```python
from build123d import *

# Parameters (mm, degrees)
F0_W     = 22.225
F0_H     = 63.5
F3_D     = 10.16
F2_R     = 19.682221
F4_DEPTH = 61.468


with BuildPart() as f1:
    # F0 (on Front) → F1 (revolve)
    with BuildSketch(Plane.XZ):
        with Locations((-11.1125, 0)):
            Rectangle(F0_W, F0_H)
    revolve(axis=Axis((0, 0, 0), (0, 0, -1)))

    # F3 (through all)
    with Locations(Plane.XY.offset(31.75)):
        with Locations((0, 0)):
            Hole(F3_D / 2)

    # F2 (on face) → F4 (cut)
    with BuildSketch(Plane.XY.offset(31.75)):
        Circle(F2_R)
    extrude(amount=-F4_DEPTH, mode=Mode.SUBTRACT)


solid = f1.part
```
Here's how the part is built. I have some questions about the finished solid (model axes, mm). A direction names the side the tool comes from. Round coordinates to 2 decimals unless told otherwise and drop trailing zeros. Loops run counter-clockwise (first coordinate to the right, second up) from the corner with the lowest first, then second, coordinate; pieces in that order, holes last.
1. Will these pins go through, and if not, where does the flat tip stop? pin 1 (8 mm diameter, centred on x = 12, z = -20, fed in from +Y); pin 2 (4 mm diameter, centred on y = -15.5, z = 18, fed in from -X); pin 3 (5 mm diameter, centred on x = 4.5, z = 2.5, fed in from -Y); pin 4 (8 mm diameter, centred on x = 0, y = 0, fed in from -Z).
Answers:
pin 1: stops at y = 20.74
pin 2: stops at x = -17.66
pin 3: stops at y = -22.13
pin 4: passes through
2. For faces 1 (the face through (-2.562, 19.515, 1.446)), 2 (the face through (5.3, 0.3, -31.75)), which set-ups out of +Z, -Z, +X, -X, +Y, -Y let a thin tool reach every point of the face, with its end or its side?
Answers:
face 1: +Z
face 2: -Z, +X, -X, +Y, -Y
3. Thinking about a two-plate mould opening in X: for faces 3 (the face through (-21.199, 6.676, 0.444)), 4 (the face through (2, -20, 31.75)), 5 (the face through (0.661, 5.037, -30.748)), which applies, released by +X, released by -X, zero draft, split by the parting line, or undercut?
Answers:
face 3: split by the parting line
face 4: zero draft
face 5: undercut
4. Suppose I cut it at D-D, the plane x = -17.5. Please give me the cut outline in (y, z), and give its area (3 significant figures).
Answers:
outline: (-13.7, -31.75) - (13.7, -31.75) - (13.7, 31.75) - (9.01, 31.75) - (9.01, -29.72) - (-9.01, -29.72) - (-9.01, 31.75) - (-13.7, 31.75) - close
area: 633 mm2
5. If I drill on probe 1 along Y at (x, z) = (0, 17) (3 decimals); probe 2 along Y at (x, z) = (0, -30.65) (3 decimals); probe 3 along Z at (x, y) = (-13.5, 4), over which ranges is the centre line in solid material (lowest first)?
Answers:
probe 1: y = -22.225 to -19.682, 19.682 to 22.225
probe 2: y = -22.225 to -5.08, 5.08 to 22.225
probe 3: z = -31.75 to -29.72
6. Suppose I cut it at C-C, the plane z = 7. Please give me the cut outline in (x, y) (3 decimals), and give its area (3 significant figures).
Answers:
outline: circle Ø44.45 at (0, 0); hole circle Ø39.364 at (0, 0)
area: 335 mm2
7. Suppose I cut it at A-A, the plane y = 0. Please give me the cut outline in (x, z) (3 decimals), and give its area (3 significant figures).
Answers:
outline: (-22.225, -31.75) - (-5.08, -31.75) - (-5.08, -29.718) - (-19.682, -29.718) - (-19.682, 31.75) - (-22.225, 31.75) - close; (5.08, -31.75) - (22.225, -31.75) - (22.225, 31.75) - (19.682, 31.75) - (19.682, -29.718) - (5.08, -29.718) - close
area: 382 mm2
